For this review, take the finished solid that the model builds, in its own axes (mm). Face numbers are marked on the shaded views. A direction names the side the tool comes from. Round coordinates to 2 decimals unless told otherwise and drop trailing zeros. Write each loop counter-clockwise with the first axis right and the second up, starting at its lowest first coordinate (ties: lowest second). Pieces come first, ordered by that corner, then holes.
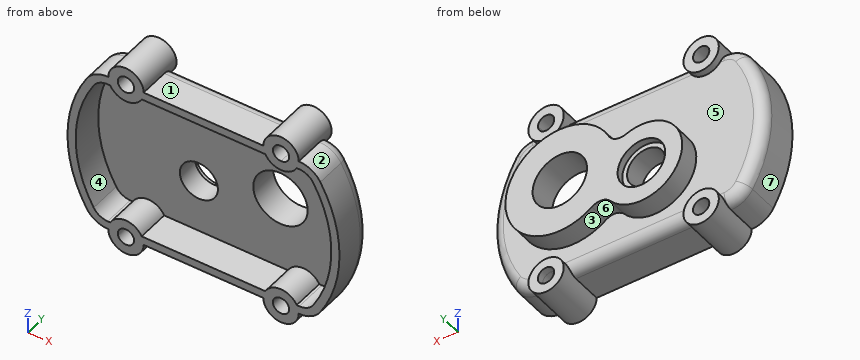
from build123d import *

# Parameters (mm, degrees)
BOSS_EXTRUDE1_DEPTH      = 30
SHELL1_T                 = -6
BOSS_EXTRUDE3_DEPTH      = 5
BOSS_EXTRUDE3_DEPTH_BACK = 30
SKETCH2_R                = 13
SKETCH2_R_2              = 6
SKETCH5_R                = 6
CUT_EXTRUDE1_DEPTH       = 35
FILLET1_R                = 8
BOSS_EXTRUDE4_DEPTH      = 15
SKETCH7_R                = 20
SKETCH7_R_2              = 14
CUT_EXTRUDE3_DEPTH       = 40
SKETCH8_R                = 17.5
CUT_EXTRUDE4_DEPTH       = 5


with BuildPart() as part:
    # Sketch1 → Boss-Extrude1 (new body)
    with BuildSketch(Plane(origin=(0, 0, 0), x_dir=(1, 0, 0), z_dir=(0, 1, 0))):
        with BuildLine():
            Line((-70.427267447, 60), (70.427267447, 60))
            ThreePointArc((70.427267447, 60), (79.316833816, 57.651696705), (85.88691152, 51.219512195))
            ThreePointArc((85.88691152, 51.219512195), (100, 0), (85.88691152, -51.219512195))
            ThreePointArc((85.88691152, -51.219512195), (79.316833816, -57.651696705), (70.427267447, -60))
            Line((70.427267447, -60), (-70.427267447, -60))
            ThreePointArc((-70.427267447, -60), (-79.316833816, -57.651696705), (-85.88691152, -51.219512195))
            ThreePointArc((-85.88691152, -51.219512195), (-100, 0), (-85.88691152, 51.219512195))
            ThreePointArc((-85.88691152, 51.219512195), (-79.316833816, 57.651696705), (-70.427267447, 60))
        make_face()
    extrude(amount=BOSS_EXTRUDE1_DEPTH)

    # Shell1
    shell1_openings = [part.faces().sort_by_distance(p)[0] for p in [
        (0, 0, 0),
    ]]
    offset(amount=SHELL1_T, openings=shell1_openings, kind=Kind.INTERSECTION)

    # Sketch2 → Boss-Extrude3 (add, two sides: drawn at the far end of the back side and taken through both)
    # profile 1 of 4: a face of its own
    with BuildSketch(Plane(origin=(0, 30, 0), x_dir=(1, 0, 0), z_dir=(0, 1, 0)).offset(-BOSS_EXTRUDE3_DEPTH_BACK)):
        with Locations(Location((57, 60, 0), (0, 0, 270))):
            Circle(SKETCH2_R)
        with Locations(Location((57, 60, 0), (0, 0, 270))):
            Circle(SKETCH2_R_2, mode=Mode.SUBTRACT)
    # profile 2 of 4: a face of its own
    with BuildSketch(Plane(origin=(0, 30, 0), x_dir=(1, 0, 0), z_dir=(0, 1, 0)).offset(-BOSS_EXTRUDE3_DEPTH_BACK)):
        with Locations((-57, 60)):
            Circle(SKETCH2_R)
        with Locations(Location((-57, 60, 0), (0, 0, 180))):
            Circle(SKETCH2_R_2, mode=Mode.SUBTRACT)
    # profile 3 of 4: a face of its own
    with BuildSketch(Plane(origin=(0, 30, 0), x_dir=(1, 0, 0), z_dir=(0, 1, 0)).offset(-BOSS_EXTRUDE3_DEPTH_BACK)):
        with Locations(Location((-57, -60, 0), (0, 0, 270))):
            Circle(SKETCH2_R)
        with Locations(Location((-57, -60, 0), (0, 0, 270))):
            Circle(SKETCH2_R_2, mode=Mode.SUBTRACT)
    # profile 4 of 4: a face of its own
    with BuildSketch(Plane(origin=(0, 30, 0), x_dir=(1, 0, 0), z_dir=(0, 1, 0)).offset(-BOSS_EXTRUDE3_DEPTH_BACK)):
        with Locations(Location((57, -60, 0), (0, 0, 180))):
            Circle(SKETCH2_R)
        with Locations((57, -60)):
            Circle(SKETCH2_R_2, mode=Mode.SUBTRACT)
    extrude(amount=BOSS_EXTRUDE3_DEPTH + BOSS_EXTRUDE3_DEPTH_BACK)

    # Sketch5 → Cut-Extrude1 (cut)
    with BuildSketch(Plane(origin=(0, 35, 0), x_dir=(1, 0, 0), z_dir=(0, 1, 0))):
        with Locations(Location((-57, 60, 0), (0, 0, 90))):
            Circle(SKETCH5_R)
        with Locations(Location((-57, -60, 0), (0, 0, 270))):
            Circle(SKETCH5_R)
        with Locations(Location((57, -60, 0), (0, 0, 90))):
            Circle(SKETCH5_R)
        with Locations(Location((57, 60, 0), (0, 0, 270))):
            Circle(SKETCH5_R)
    extrude(amount=-CUT_EXTRUDE1_DEPTH, mode=Mode.SUBTRACT)

    # Fillet1
    # the kernel refuses this fillet: 8 mm, written as the material it takes off along each edge
    with BuildSketch(Plane(origin=(-70.427267447, 30, -42), x_dir=(-0.858869115202879, 0, -0.5121951219512186), z_dir=(-0.5121951219512186, 0, 0.858869115202879))) as fillet1_piece_1:
        with BuildLine():
            CenterArc((18 - FILLET1_R, FILLET1_R), FILLET1_R, 270, 90)
            Line((18 - FILLET1_R, 0), (18, 0))
            Line((18, 0), (18, FILLET1_R))
        make_face()
    revolve(axis=Axis((-70.427267447, 30, -42), (0, -1, 0)), revolution_arc=59.189843357, mode=Mode.SUBTRACT)
    with BuildSketch(Plane(origin=(70.427267447, 30, 60), x_dir=(0, 0, -1), z_dir=(-1, 0, 0))) as fillet1_piece_2_section:
        with BuildLine():
            CenterArc((FILLET1_R, FILLET1_R), FILLET1_R, 180, 90)
            Line((0, FILLET1_R), (0, 0))
            Line((0, 0), (FILLET1_R, 0))
        make_face()
    fillet1_piece_2 = extrude(amount=20.427267447, mode=Mode.PRIVATE)
    fillet1_piece_2 = fillet1_piece_2 - Plane(origin=(57, 28.58355389, 60), x_dir=(-1, 0, 0), z_dir=(0, 1, 0)) * Cylinder(13, 73, mode=Mode.PRIVATE)
    add(fillet1_piece_2, mode=Mode.SUBTRACT)
    with BuildSketch(Plane(origin=(0, 30, 0), x_dir=(-0.8588691152028786, 0, 0.5121951219512192), z_dir=(0.5121951219512192, 0, 0.8588691152028786))) as fillet1_piece_3:
        with BuildLine():
            CenterArc((100 - FILLET1_R, FILLET1_R), FILLET1_R, 270, 90)
            Line((100 - FILLET1_R, 0), (100, 0))
            Line((100, 0), (100, FILLET1_R))
        make_face()
    revolve(axis=Axis((0, 30, 0), (0, -1, 0)), revolution_arc=61.620313286, mode=Mode.SUBTRACT)
    with BuildSketch(Plane(origin=(-70.427267447, 30, 42), x_dir=(0, 0, 1), z_dir=(1, 0, 0))) as fillet1_piece_4:
        with BuildLine():
            CenterArc((18 - FILLET1_R, FILLET1_R), FILLET1_R, 270, 90)
            Line((18 - FILLET1_R, 0), (18, 0))
            Line((18, 0), (18, FILLET1_R))
        make_face()
    revolve(axis=Axis((-70.427267447, 30, 42), (0, -1, 0)), revolution_arc=59.189843357, mode=Mode.SUBTRACT)
    with BuildSketch(Plane(origin=(-50, 30, 60), x_dir=(0, 0, -1), z_dir=(-1, 0, 0))) as fillet1_piece_5_section:
        with BuildLine():
            CenterArc((FILLET1_R, FILLET1_R), FILLET1_R, 180, 90)
            Line((0, FILLET1_R), (0, 0))
            Line((0, 0), (FILLET1_R, 0))
        make_face()
    fillet1_piece_5 = extrude(amount=20.427267447, mode=Mode.PRIVATE)
    fillet1_piece_5 = fillet1_piece_5 - Plane(origin=(-57, 28.583553668, 60), x_dir=(0, 0, 1), z_dir=(0, 1, 0)) * Cylinder(13, 73, mode=Mode.PRIVATE)
    add(fillet1_piece_5, mode=Mode.SUBTRACT)
    with BuildSketch(Plane(origin=(70.427267447, 30, 42), x_dir=(0.8588691152028791, 0, 0.5121951219512185), z_dir=(0.5121951219512185, 0, -0.8588691152028791))) as fillet1_piece_6:
        with BuildLine():
            CenterArc((18 - FILLET1_R, FILLET1_R), FILLET1_R, 270, 90)
            Line((18, FILLET1_R), (18, 0))
            Line((18, 0), (18 - FILLET1_R, 0))
        make_face()
    revolve(axis=Axis((70.427267447, 30, 42), (0, -1, 0)), revolution_arc=59.189843357, mode=Mode.SUBTRACT)
    with BuildSketch(Plane(origin=(0, 30, 0), x_dir=(0.8588691152028793, 0, -0.5121951219512181), z_dir=(-0.5121951219512181, 0, -0.8588691152028793))) as fillet1_piece_7:
        with BuildLine():
            CenterArc((100 - FILLET1_R, FILLET1_R), FILLET1_R, 270, 90)
            Line((100, FILLET1_R), (100, 0))
            Line((100, 0), (100 - FILLET1_R, 0))
        make_face()
    revolve(axis=Axis((0, 30, 0), (0, -1, 0)), revolution_arc=61.620313286, mode=Mode.SUBTRACT)
    with BuildSketch(Plane(origin=(70.427267447, 30, -42), x_dir=(0, 0, -1), z_dir=(-1, 0, 0))) as fillet1_piece_8:
        with BuildLine():
            CenterArc((18 - FILLET1_R, FILLET1_R), FILLET1_R, 270, 90)
            Line((18, FILLET1_R), (18, 0))
            Line((18, 0), (18 - FILLET1_R, 0))
        make_face()
    revolve(axis=Axis((70.427267447, 30, -42), (0, -1, 0)), revolution_arc=59.189843357, mode=Mode.SUBTRACT)
    with BuildSketch(Plane(origin=(-64, 30, -60), x_dir=(0, 0, 1), z_dir=(1, 0, 0))) as fillet1_piece_9_section:
        with BuildLine():
            CenterArc((FILLET1_R, FILLET1_R), FILLET1_R, 180, 90)
            Line((0, FILLET1_R), (0, 0))
            Line((0, 0), (FILLET1_R, 0))
        make_face()
    fillet1_piece_9 = extrude(amount=128, mode=Mode.PRIVATE)
    fillet1_piece_9 = fillet1_piece_9 - Plane(origin=(-57, 28.21841699, -60), x_dir=(1, 0, 0), z_dir=(0, 1, 0)) * Cylinder(13, 288, mode=Mode.PRIVATE)
    fillet1_piece_9 = fillet1_piece_9 - Plane(origin=(57, 28.21841699, -60), x_dir=(0, 0, 1), z_dir=(0, 1, 0)) * Cylinder(13, 288, mode=Mode.PRIVATE)
    add(fillet1_piece_9, mode=Mode.SUBTRACT)
    with BuildSketch(Plane(origin=(-70.427267447, 30, -60), x_dir=(0, 0, 1), z_dir=(1, 0, 0))) as fillet1_piece_10_section:
        with BuildLine():
            CenterArc((FILLET1_R, FILLET1_R), FILLET1_R, 180, 90)
            Line((0, FILLET1_R), (0, 0))
            Line((0, 0), (FILLET1_R, 0))
        make_face()
    fillet1_piece_10 = extrude(amount=20.427267447, mode=Mode.PRIVATE)
    fillet1_piece_10 = fillet1_piece_10 - Plane(origin=(-57, 28.583553949, -60), x_dir=(1, 0, 0), z_dir=(0, 1, 0)) * Cylinder(13, 73, mode=Mode.PRIVATE)
    add(fillet1_piece_10, mode=Mode.SUBTRACT)
    with BuildSketch(Plane(origin=(50, 30, -60), x_dir=(0, 0, 1), z_dir=(1, 0, 0))) as fillet1_piece_11_section:
        with BuildLine():
            CenterArc((FILLET1_R, FILLET1_R), FILLET1_R, 180, 90)
            Line((0, FILLET1_R), (0, 0))
            Line((0, 0), (FILLET1_R, 0))
        make_face()
    fillet1_piece_11 = extrude(amount=20.427267447, mode=Mode.PRIVATE)
    fillet1_piece_11 = fillet1_piece_11 - Plane(origin=(57, 28.583553668, -60), x_dir=(0, 0, 1), z_dir=(0, 1, 0)) * Cylinder(13, 73, mode=Mode.PRIVATE)
    add(fillet1_piece_11, mode=Mode.SUBTRACT)
    with BuildSketch(Plane(origin=(64, 30, 60), x_dir=(0, 0, -1), z_dir=(-1, 0, 0))) as fillet1_piece_12_section:
        with BuildLine():
            CenterArc((FILLET1_R, FILLET1_R), FILLET1_R, 180, 90)
            Line((0, FILLET1_R), (0, 0))
            Line((0, 0), (FILLET1_R, 0))
        make_face()
    fillet1_piece_12 = extrude(amount=128, mode=Mode.PRIVATE)
    fillet1_piece_12 = fillet1_piece_12 - Plane(origin=(-57, 28.21841699, 60), x_dir=(0, 0, 1), z_dir=(0, 1, 0)) * Cylinder(13, 288, mode=Mode.PRIVATE)
    fillet1_piece_12 = fillet1_piece_12 - Plane(origin=(57, 28.21841699, 60), x_dir=(-1, 0, 0), z_dir=(0, 1, 0)) * Cylinder(13, 288, mode=Mode.PRIVATE)
    add(fillet1_piece_12, mode=Mode.SUBTRACT)

    # Sketch6 → Boss-Extrude4 (add)
    with BuildSketch(Plane(origin=(0, 30, 0), x_dir=(1, 0, 0), z_dir=(0, 1, 0))):
        with BuildLine():
            ThreePointArc((4.207246611, -17.857177964), (78.857900978, -9.4901808), (16.468229876, 32.345877555))
            ThreePointArc((16.468229876, 32.345877555), (9.380607501, 30.505174816), (2.938965509, 33.987677645))
            ThreePointArc((2.938965509, 33.987677645), (-49.143425733, 21.771305347), (-8.555706302, -13.077686905))
            ThreePointArc((-8.555706302, -13.077686905), (-1.233963888, -12.95658557), (4.207246611, -17.857177964))
        make_face()
    extrude(amount=BOSS_EXTRUDE4_DEPTH)

    # Sketch7 → Cut-Extrude3 (cut)
    with BuildSketch(Plane(origin=(0, 45, 0), x_dir=(1, 0, 0), z_dir=(0, 1, 0))):
        with Locations(Location((40, 0, 0), (0, 0, 270))):
            Circle(SKETCH7_R)
        with Locations(Location((-20, 14.653669747, 0), (0, 0, 270))):
            Circle(SKETCH7_R_2)
    extrude(amount=-CUT_EXTRUDE3_DEPTH, mode=Mode.SUBTRACT)

    # Sketch8 → Cut-Extrude4 (cut)
    with BuildSketch(Plane(origin=(0, 45, 0), x_dir=(1, 0, 0), z_dir=(0, 1, 0))):
        with Locations(Location((-20, 14.653669747, 0), (0, 0, 270))):
            Circle(SKETCH8_R)
    extrude(amount=-CUT_EXTRUDE4_DEPTH, mode=Mode.SUBTRACT)


solid = part.part
(1) For pin 1 Ø1 at (x, z) = (-55, -23.5) entering from +Y; pin 2 Ø6 at (x, z) = (71, 13) entering from -Y; pin 3 Ø1.5 at (x, y) = (20, 11.5) entering from -Z; pin 4 Ø9.5 at (x, z) = (-57, 60) entering from -Y, all flat-tipped, find the tip position at first contact; note any pin that passes through.
Geometry check:
pin 1: stops at y = 30
pin 2: stops at y = 24
pin 3: stops at z = -60
pin 4: passes through
(2) We need section B-B, the plane x = -57. Give the boundary of the cut face in (y, z), and give its area (3 significant figures).
Geometry check:
outline: (0, -73) - (35, -73) - (35, -66) - (0, -66) - close; (0, -54) - (35, -54) - (35, -47) - (30, -47) - (30, 47) - (35, 47) - (35, 54) - (0, 54) - (0, 47) - (24, 47) - (24, -47) - (0, -47) - close; (0, 66) - (35, 66) - (35, 73) - (0, 73) - close
area: 1,540 mm2
(3) We need section A-A, the plane x = 40. Give the boundary of the cut face in (y, z).
Geometry check:
outline: (0, -60) - (22, -60) arc R8 ccw to (30, -52) - (30, -40) - (45, -40) - (45, -20) - (24, -20) - (24, -54) - (0, -54) - close; (0, 54) - (24, 54) - (24, 20) - (45, 20) - (45, 40) - (30, 40) - (30, 52) arc R8 ccw to (22, 60) - (0, 60) - close
(4) For the marked faces 1, 2, 3 and 4, list the 3-axis set-ups (+Z, -Z, +X, -X, +Y, -Y) from which the entire face can be reached by the end or side of a thin tool; tool diameter is ignored.
Geometry check:
face 1: +Z, +Y, -Y
face 2: +Z, +X, +Y, -Y
face 3: +Y
face 4: -Y
(5) For line 1 along X through (y, z) = (25.5, 60); line 2 along Z through (x, y) = (57, 8); line 3 along Z through (x, y) = (42, 10), list the stretches that pass through material, from the lowest coordinate up.
Geometry check:
line 1: x = -70 to -63, -51 to -44, 44 to 51, 63 to 70
line 2: z = -73 to -66, -54 to -47, 47 to 54, 66 to 73
line 3: z = -60 to -54, 54 to 60
(6) We need section C-C, the plane z = -15.5. State how many separate pieces and enclosed holes the cut face has, and give its area (3 significant figures).
Geometry check:
separate pieces: 3
enclosed holes: 0
area: 2,200 mm2
(7) Mouldability with a two-part tool opening along Z and no side actions: class the marked faces 5, 6 and 7 as pulls with the +Z half, pulls with the -Z half, needs draft (parallel to the pull), parting line crosses it, or undercut.
Geometry check:
face 5: undercut
face 6: pulls with the -Z half
face 7: parting line crosses it
